```python
from build123d import *

# Parameters (mm, degrees)
F0_R          = 6
F1_DEPTH      = 10
F2_R          = 10
F3_DEPTH      = 8
F3_DEPTH_BACK = 8


with BuildPart() as f1:
    # F0 (on Top) → F1 (new body)
    with BuildSketch(Plane.XY):
        with BuildLine():
            ThreePointArc((50.720724, 17.985565), (30.362055, 23.224109), (13.956018, 36.367918))
            ThreePointArc((13.956018, 36.367918), (-6.032896, 41.958896), (-18, 25))
            Line((-18, 25), (-18, 0))
            Line((-18, 0), (-18, -25))
            ThreePointArc((-18, -25), (-6.032896, -41.958896), (13.956018, -36.367918))
            ThreePointArc((13.956018, -36.367918), (30.362055, -23.224109), (50.720724, -17.985565))
            ThreePointArc((50.720724, -17.985565), (62.980236, -12.470505), (68, 0))
            ThreePointArc((68, 0), (62.980236, 12.470505), (50.720724, 17.985565))
        make_face()
        with Locations((0, -25)):
            Circle(F0_R, mode=Mode.SUBTRACT)
        with Locations((0, 25)):
            Circle(F0_R, mode=Mode.SUBTRACT)
        with BuildLine():
            ThreePointArc((44, 0), (50, 6), (56, 0))
            ThreePointArc((56, 0), (50, -6), (44, 0))
        make_face(mode=Mode.SUBTRACT)
    extrude(amount=F1_DEPTH)

    # F2 (on Front) → F3 (join, two sides)
    with BuildSketch(Plane.XZ) as f3_sk:
        with BuildLine():
            Line((-60, 0), (0, 0))
            Line((0, 0), (34.021274, 0))
            Line((34.021274, 0), (34.021274, 10))
            ThreePointArc((34.021274, 10), (-8.487228, 17.449895), (-45.928789, 38.911565))
            ThreePointArc((-45.928789, 38.911565), (-80.688818, 29.481496), (-60, 0))
        make_face()
        with Locations((-60, 22)):
            Circle(F2_R, mode=Mode.SUBTRACT)
    extrude(amount=F3_DEPTH)
    extrude(f3_sk.sketch, amount=-F3_DEPTH_BACK)


solid = f1.part
```
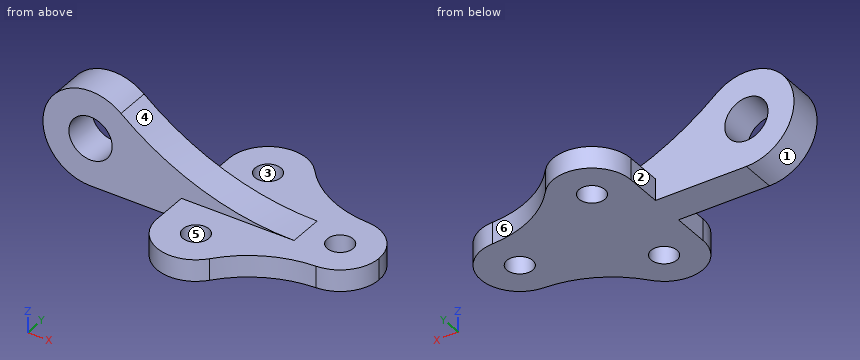
Read the model definition and answer for the solid it produces. Units are mm, in the model's axes. Face numbers are marked on the shaded views. A direction names the side the tool comes from. Give positions to 0.01 mm unless a question says otherwise; leave off trailing zeros. Order: outer loops, then holes, each group sorted by start corner. A loop starts at its lowest first (then second) coordinate and runs counter-clockwise, first axis right, second up.
(1) Find section A-A (z = 22). Give the vertices of the cut face in (x, y).
(2) Find section D-D (x = 16.5). Give the vertices of the cut face in (y, z).
(3) Find section B-B (y = -22). Give the vertices of the cut face in (x, z), plus the area to 3 significant figures.
(4) For a pull along Y with two mould halves and no side action, classify the marked faces 3, 4, 5 and 6 as released by +Y, released by -Y, zero draft, split by the parting line, or undercut.
(5) For the marked faces 1 and 2, determine the directions among +Z, -Z, +X, -X, +Y, -Y from which every point of the face is accessible in a straight line to the end or side of a thin tool.
(6) Given pin 1 (4 mm diameter, centred on x = -12.5, z = 8.5, fed in from -Y); pin 2 (1.5 mm diameter, centred on x = 4.5, y = 1.5, fed in from +Z); pin 3 (1.5 mm diameter, centred on x = 6.5, z = 10.5, fed in from -Y), each flat-ended and moving along its own axis, determine where each tip first touches the part or whether it passes through.
(7) Find section C-C (x = -3). Give the vertices of the cut face in (y, z).
(8) Straight lines are drawn through the part: L1, parallel to Y at x = 0, z = 5.75; L2, parallel to Z at x = -60, y = 0; L3, parallel to Y at x = -70.5, z = 9. For each, find the intervals that lie inside material, in ascending order.
Result sheet:
1. outline: (-82, -8) - (-70, -8) - (-70, 8) - (-82, 8) - close; (-50, -8) - (-19.42, -8) - (-19.42, 8) - (-50, 8) - close
2. outline: (-33.48, 0) - (33.48, 0) - (33.48, 10) - (8, 10) - (8, 11.23) - (-8, 11.23) - (-8, 10) - (-33.48, 10) - close
3. outline: (-18, 0) - (-5.2, 0) - (-5.2, 10) - (-18, 10) - close; (5.2, 0) - (33, 0) - (33, 10) - (5.2, 10) - close
3. area: 406 mm2
4. face 3: undercut
4. face 4: zero draft
4. face 5: undercut
4. face 6: released by +Y
5. face 1: +Y, -Y
5. face 2: +Z, -Z, -X, +Y
6. pin 1: stops at y = -39.62
6. pin 2: stops at z = 13.72
6. pin 3: stops at y = -41.99
7. outline: (-42.75, 0) - (-30.2, 0) - (-30.2, 10) - (-42.75, 10) - close; (-19.8, 0) - (19.8, 0) - (19.8, 10) - (8, 10) - (8, 15.61) - (-8, 15.61) - (-8, 10) - (-19.8, 10) - close; (30.2, 0) - (42.75, 0) - (42.75, 10) - (30.2, 10) - close
8. L1: y = -43 to -31, -19 to 19, 31 to 43
8. L2: z = 0 to 12, 32 to 44
8. L3: y = -8 to 8
